from build123d import *

# Parameters (mm, degrees)
SKETCH1_R           = 44
BOSS_EXTRUDE1_DEPTH = 150
BOSS_EXTRUDE2_DEPTH = 12
SKETCH5_R           = 6.5
CUT_EXTRUDE3_DEPTH  = 80
SKETCH6_R           = 35
CUT_EXTRUDE4_DEPTH  = 147
SKETCH7_R           = 25.5
CUT_EXTRUDE5_DEPTH  = 67


with BuildPart() as part:
    # Sketch1 → Boss-Extrude1 (new body)
    with BuildSketch(Plane(origin=(0, 0, 0), x_dir=(0, 0, -1), z_dir=(1, 0, 0))):
        Circle(SKETCH1_R)
    extrude(amount=BOSS_EXTRUDE1_DEPTH)

    # Sketch2 → Boss-Extrude2 (add)
    with BuildSketch(Plane(origin=(150, 0, 0), x_dir=(0, 0, -1), z_dir=(1, 0, 0))):
        with BuildLine():
            Line((-25.925925926, 42.753319928), (-75.277777778, 12.825995978))
            ThreePointArc((-75.277777778, 12.825995978), (-82.5, 0), (-75.277777778, -12.825995978))
            Line((-75.277777778, -12.825995978), (-25.925925926, -42.753319928))
            ThreePointArc((-25.925925926, -42.753319928), (0, -50), (25.925925926, -42.753319928))
            Line((25.925925926, -42.753319928), (75.277777778, -12.825995978))
            ThreePointArc((75.277777778, -12.825995978), (82.5, 0), (75.277777778, 12.825995978))
            Line((75.277777778, 12.825995978), (25.925925926, 42.753319928))
            ThreePointArc((25.925925926, 42.753319928), (0, 50), (-25.925925926, 42.753319928))
        make_face()
    extrude(amount=BOSS_EXTRUDE2_DEPTH)

    # Sketch5 → Cut-Extrude3 (cut)
    with BuildSketch(Plane(origin=(162, 0, 0), x_dir=(0, 0, -1), z_dir=(1, 0, 0))):
        with Locations((67.5, 0)):
            Circle(SKETCH5_R)
        with Locations((-67.5, 0)):
            Circle(SKETCH5_R)
    extrude(amount=-CUT_EXTRUDE3_DEPTH, mode=Mode.SUBTRACT)

    # Sketch6 → Cut-Extrude4 (cut)
    with BuildSketch(Plane(origin=(162, 0, 0), x_dir=(0, 0, -1), z_dir=(1, 0, 0))):
        Circle(SKETCH6_R)
    extrude(amount=-CUT_EXTRUDE4_DEPTH, mode=Mode.SUBTRACT)

    # Sketch7 → Cut-Extrude5 (cut)
    with BuildSketch(Plane.ZY):
        Circle(SKETCH7_R)
    extrude(amount=-CUT_EXTRUDE5_DEPTH, mode=Mode.SUBTRACT)


solid = part.part
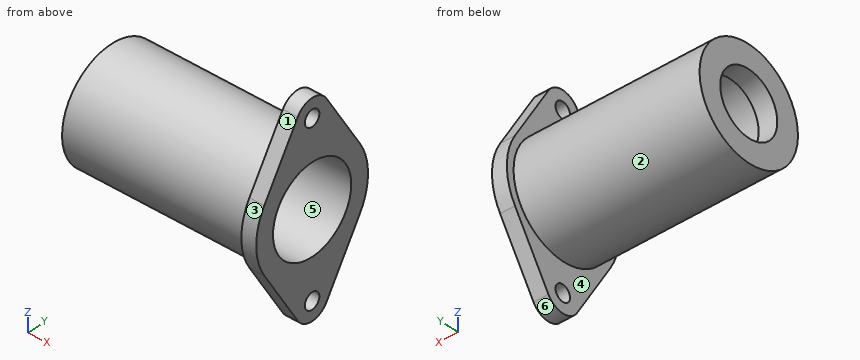
Build history of the part. All positions in model axes, mm. Face numbers are marked on the shaded views. A direction names the side the tool comes from. Coordinates: 2 decimals unless noted, no trailing zeros. Order: outer loops, then holes, each group sorted by start corner. A loop starts at its lowest first (then second) coordinate and runs counter-clockwise, first axis right, second up. Notation, with made-up numbers: (69, 46) - (93, 46) arc R18 ccw to (93, 65) - close; hole circle Ø2 at (-33, -23.75). An arc over 180 degrees is marked (long way). Put each result on its own line as item: value.
1. Pull direction Z, two halves, no side cores. Call the marked faces 3, 4, 5 and 6: pulls with the +Z half, pulls with the -Z half, needs draft (parallel to the pull), parting line crosses it, or undercut.
Answer sheet:
face 3: parting line crosses it
face 4: needs draft
face 5: undercut
face 6: pulls with the -Z half
2. Tool access for the marked faces 1 and 2: list every direction of +Z, -Z, +X, -X, +Y, -Y with a clear straight run to the whole face (end or side of a thin tool).
Answer sheet:
face 1: +Z, +X, -X, -Y
face 2: -X
3. Saw through at A-A (y = 23). Write the cut outline in (x, z), and give its area (3 significant figures).
Answer sheet:
outline: (0, -37.51) - (150, -37.51) - (150, -58.5) - (162, -58.5) - (162, -26.38) - (15, -26.38) - (15, -11.01) - (0, -11.01) - close; (0, 11.01) - (15, 11.01) - (15, 26.38) - (162, 26.38) - (162, 58.5) - (150, 58.5) - (150, 37.51) - (0, 37.51) - close
area: 4,570 mm^2
4. Saw through at B-B (z = 0). Write the cut outline in (x, y).
Answer sheet:
outline: (0, -44) - (150, -44) - (150, -50) - (162, -50) - (162, -35) - (15, -35) - (15, -25.5) - (0, -25.5) - close; (0, 25.5) - (15, 25.5) - (15, 35) - (162, 35) - (162, 50) - (150, 50) - (150, 44) - (0, 44) - close
5. Saw through at D-D (x = 145.5). Write the cut outline in (y, z).
Answer sheet:
outline: circle Ø88 at (0, 0); hole circle Ø70 at (0, 0)
6. Saw through at C-C (y = 0). Write the cut outline in (x, z).
Answer sheet:
outline: (0, -44) - (150, -44) - (150, -61) - (162, -61) - (162, -35) - (15, -35) - (15, -25.5) - (0, -25.5) - close; (0, 25.5) - (15, 25.5) - (15, 35) - (162, 35) - (162, 61) - (150, 61) - (150, 44) - (0, 44) - close; (150, -82.5) - (162, -82.5) - (162, -74) - (150, -74) - close; (150, 74) - (162, 74) - (162, 82.5) - (150, 82.5) - close
7. Probe line 1 along Y through (x, z) = (136, -1.5); line 2 along X through (y, z) = (-15.5, 59); line 3 along Z through (x, y) = (146, -21). List the from-to ranges inside material, lowest first. Write a range as [from, to].
Answer sheet:
line 1: y = [-43.97, -34.97], [34.97, 43.97]
line 2: x = [150, 162]
line 3: z = [-38.67, -28], [28, 38.67]
8. Drop flat-ended pins along their axis: P1, Ø10, axis at x = 111, z = -36, coming from the +Y side (3 decimals); P2, Ø1, axis at x = 79.5, z = 3.5, coming from the +Y side; P3, Ø8, axis at x = 28, y = -37, coming from the +Z side. Give the stop position or say it passes through.
Answer sheet:
P1: stops at y = 31.225
P2: stops at y = 43.9
P3: stops at z = 29.1
